Autodesk Fusion 360 part; units mm, degrees
sketch "Skizze1" plane through (0, 0, 0) normal (0, 0, 1) x (1, 0, 0)
  line L0 (-50, 50) -> (0, 50)
  line L1 (0, 50) -> (0, 0)
  line L2 (0, 0) -> (-50, 0)
  line L3 (-50, 0) -> (-50, 50)
  line L4 (-50, 25) -> (0, 25) construction
  line L5 (-25, 50) -> (-25, 0) construction
  circle A0 centre (-25, 25) radius 16.5
  circle A1 centre (-8.0294, 8.0294) radius 3.55
  line L6 (-50, 50) -> (0, 0) construction
  line L7 (0, 50) -> (-50, 0) construction
  circle A2 centre (-43.3848, 43.3848) radius 1.9
  circle A3 centre (-6.6152, 43.3848) radius 1.9
  circle A4 centre (-43.3848, 6.6152) radius 1.9
  line L8 (-6.8665, 50) -> (0, 43.1335)
  line L9 (-50, 6.8665) -> (-43.1335, 0)
  line L10 (-43.1335, 50) -> (-50, 43.1335)
  line L11 (0, 6.8665) -> (-6.8665, 0)
  line L12 (-8.0294, 16.5147) -> (-16.5147, 8.0294) construction
  line L13 (-16.5147, 8.0294) -> (-8.0294, -0.4558) construction
  line L14 (-8.0294, -0.4558) -> (0.4558, 8.0294) construction
  line L15 (0.4558, 8.0294) -> (-8.0294, 16.5147) construction
  line L16 (-8.0294, 16.5147) -> (-8.0294, -0.4558) construction
  point P0 (-8.0294, 8.0294)
  point P1 (-8.0294, 8.0294)
  dimension "d3" = 33
  dimension "d4" = 7.1
  dimension "d6" = 3.8
  dimension "d7" = 26
  dimension "d8" = 26
  dimension "d9" = 26
  dimension "d42" = 50
  dimension "d43" = 50
  dimension "d44" = 61
  dimension "d45" = 61
  dimension "d46" = 12
  dimension "d47" = 12
  dimension "d54" = 6.5
extrude "Extrusion1" add sketch "Skizze1" along normal blind 3 contours L0 L1 L2 L3 L8 L9 L10 L11
chamfer "Fase1" distance 0.8 angle 45 8 edges at (-25, 0, 3) (-46.5668, 3.4332, 3) (-50, 25, 3) (-46.5668, 46.5668, 3) (-25, 50, 3) (-3.4332, 46.5668, 3) (0, 25, 3) (-3.4332, 3.4332, 3)
chamfer "Fase3" distance 2 distance2 1 1 edges at (-40.3834, 30.9667, 3) measured on face at (-24.589, 46.618, 3)
sketch "Skizze2" plane through (0, 0, 0) normal (0, 0, -1) x (1, 0, 0)
  circle A0 centre (-25, -25) radius 16.5
  circle A1 centre (-43.3848, -43.3848) radius 1.9
  circle A2 centre (-43.3848, -6.6152) radius 1.9
  circle A3 centre (-8.0294, -8.0294) radius 3.55
  circle A4 centre (-6.6152, -43.3848) radius 1.9
  line L0 (-50, -43.1335) -> (-43.1335, -50)
  line L1 (-43.1335, -50) -> (-6.8665, -50)
  line L2 (-6.8665, -50) -> (0, -43.1335)
  line L3 (0, -43.1335) -> (0, -6.8665)
  line L4 (0, -6.8665) -> (-6.8665, 0)
  line L5 (-6.8665, 0) -> (-43.1335, 0)
  line L6 (-43.1335, 0) -> (-50, -6.8665)
  line L7 (-50, -6.8665) -> (-50, -43.1335)
  circle A5 centre (-25, -25) radius 18.35
  line L8 (-14.75, -9.7796) -> (-17.9, -3.55)
  line L9 (-17.9, -3.55) -> (-32.1, -3.55)
  line L10 (-32.1, -3.55) -> (-35.25, -9.7796)
  line L11 (-25, -25) -> (-25, 4.0219) construction
  dimension "d18" = 36.7
  dimension "d19" = 21.45
  dimension "d20" = 20.5
  dimension "d21" = 14.2
extrude "Extrusion2" cut sketch "Skizze2" against normal blind 1.5 contours A5 | A5 L8 L9 L10
sketch "Skizze3" plane through (0, 0, 0) normal (0, -1, 0) x (1, 0, 0)
  line L0 (-6.8665, 2.2) -> (-43.1335, 2.2)
  line L1 (-43.1335, 2.2) -> (-43.1335, 0)
  line L2 (-43.1335, 0) -> (-6.8665, 0)
  line L3 (-6.8665, 0) -> (-6.8665, 2.2)
  line L4 (-41.5, 1.5) -> (-8.5, 1.5)
  line L5 (-41.5, 2) -> (-8.5, 2)
  line L6 (-25, 1.5) -> (-25, -10) construction
  line L7 (-22.9, -6.8) -> (-27.1, -6.8)
  line L8 (-22.9, -0.8) -> (-27.1, -0.8)
  arc A0 (-27.1, -0.8) -> (-27.1, -6.8) centre (-27.1, -3.8) ccw
  arc A1 (-22.9, -6.8) -> (-22.9, -0.8) centre (-22.9, -3.8) ccw
  line L9 (-19.9, -3.8) -> (-30.1, -3.8) construction
  line L10 (-25, -5.5) -> (-25, -2.1) construction
  line L11 (-22.9, -6.8) -> (-19.9, -6.8)
  line L12 (-19.9, -6.8) -> (-19.9, -3.8)
  line L13 (-27.1, -6.8) -> (-30.1, -6.8)
  line L14 (-30.1, -6.8) -> (-30.1, -3.8)
  line L15 (-30.1, -6.8) -> (-19.9, -6.8)
  line L16 (-19.9, -6.8) -> (-19.9, -8.8)
  line L17 (-19.9, -8.8) -> (-30.1, -8.8)
  line L18 (-30.1, -8.8) -> (-30.1, -6.8)
  point P0 (-25, -2.1)
  point P1 (-25, -5.5)
  point P2 (-25, -3.8)
  point P3 (-25, -3.8)
  dimension "d24" = 3.6
  dimension "d25" = 7
  dimension "d27" = 6
  dimension "d31" = 10.2
  dimension "d53" = 2
extrude "Extrusion3" add 1 faces at (-47.7677, 25.4366, 0) along direction (0, 0, -1) blind 7
extrude "Extrusion4" cut sketch "Skizze3" against normal up to surface (3.55 mm away) contours L7 L11 L13 L15 L16 L17 L18 | L7 L8 A0 A1 L15 | A1 L11 L12 L15 | A0 L13 L14 L15
sketch "Skizze4" plane through (0, 0, -7) normal (0, 0, -1) x (1, 0, 0)
  circle A0 centre (-43.3848, -43.3848) radius 1.9
  circle A1 centre (-6.6152, -43.3848) radius 1.9
  arc A2 (-35.25, -9.7796) -> (-14.75, -9.7796) centre (-25, -25) ccw
  arc A3 (-35.25, -9.7796) -> (-14.75, -9.7796) centre (-25, -25) ccw
  circle A4 centre (-8.0294, -8.0294) radius 3.55
  circle A5 centre (-8.0294, -8.0294) radius 3.55
  circle A6 centre (-43.3848, -6.6152) radius 1.9
  circle A7 centre (-8.0294, -8.0294) radius 3.5
  circle A8 centre (-8.0294, -8.0294) radius 5
  circle A9 centre (-6.6152, -43.3848) radius 1.1
  circle A10 centre (-6.6152, -43.3848) radius 3
  circle A11 centre (-43.3848, -43.3848) radius 1.1
  circle A12 centre (-43.3848, -43.3848) radius 3
  circle A13 centre (-43.3848, -6.6152) radius 1.1
  circle A14 centre (-43.3848, -6.6152) radius 3
  circle A15 centre (-43.3848, -43.3848) radius 1.9
  circle A16 centre (-6.6152, -43.3848) radius 1.9
  circle A17 centre (-43.3848, -6.6152) radius 1.9
  dimension "d49" = 6
  dimension "d50" = 10
extrude "Extrusion5" cut sketch "Skizze4" against normal blind 4 contours A10 | A12 | A14
extrude "Extrusion6" cut sketch "Skizze4" against normal blind 3 contours A8
sketch "Skizze5" plane through (0, 0, 3) normal (0, 0, 1) x (-1, 0, 0)
  line L0 (7.1979, -49.2) -> (42.8021, -49.2)
  line L1 (42.8021, -49.2) -> (49.2, -42.8021)
  line L2 (49.2, -42.8021) -> (49.2, -7.1979)
  line L3 (49.2, -7.1979) -> (42.8021, -0.8)
  line L4 (42.8021, -0.8) -> (7.1979, -0.8)
  line L5 (7.1979, -0.8) -> (0.8, -7.1979)
  line L6 (0.8, -7.1979) -> (0.8, -42.8021)
  line L7 (0.8, -42.8021) -> (7.1979, -49.2)
  circle A0 centre (43.3848, -43.3848) radius 1.9
  circle A1 centre (43.3848, -6.6152) radius 1.9
  circle A2 centre (6.6152, -43.3848) radius 1.9
  circle A3 centre (8.0294, -8.0294) radius 3.55
  circle A4 centre (25, -25) radius 18.5
  circle A5 centre (6.6152, -43.3848) radius 1.9
  circle A6 centre (6.6152, -43.3848) radius 1.9
  circle A7 centre (43.3848, -43.3848) radius 1.9
  circle A8 centre (43.3848, -43.3848) radius 1.9
  circle A9 centre (43.3848, -6.6152) radius 1.9
  circle A10 centre (43.3848, -6.6152) radius 1.9
  circle A11 centre (43.3848, -43.3848) radius 3.5
  circle A12 centre (43.3848, -6.6152) radius 3.5
  circle A13 centre (6.6152, -43.3848) radius 3.5
  dimension "d55" = 7
extrude "Extrusion7" cut sketch "Skizze5" against normal blind 2.4 contours A11 | A12 | A13
sketch "Skizze6" plane through (0, 0, -7) normal (0, 0, -1) x (1, 0, 0)
  circle A0 centre (-8.0294, -8.0294) radius 5
  line L0 (-30.1, -3.55) -> (-30.1, 0)
  line L1 (-30.1, 0) -> (-43.1335, 0)
  line L2 (-43.1335, 0) -> (-50, -6.8665)
  line L3 (-50, -6.8665) -> (-50, -43.1335)
  line L4 (-50, -43.1335) -> (-43.1335, -50)
  line L5 (-43.1335, -50) -> (-6.8665, -50)
  line L6 (-6.8665, -50) -> (0, -43.1335)
  line L7 (0, -43.1335) -> (0, -6.8665)
  line L8 (0, -6.8665) -> (-6.8665, 0)
  line L9 (-6.8665, 0) -> (-19.9, 0)
  line L10 (-19.9, 0) -> (-19.9, -3.55)
  line L11 (-19.9, -3.55) -> (-17.9, -3.55)
  line L12 (-17.9, -3.55) -> (-14.75, -9.7796)
  arc A1 (-35.25, -9.7796) -> (-14.75, -9.7796) centre (-25, -25) ccw
  line L13 (-35.25, -9.7796) -> (-32.1, -3.55)
  line L14 (-32.1, -3.55) -> (-30.1, -3.55)
  circle A2 centre (-6.6152, -43.3848) radius 3
  circle A3 centre (-43.3848, -43.3848) radius 3
  circle A4 centre (-43.3848, -6.6152) radius 3
  circle A5 centre (-6.6152, -43.3848) radius 3
  circle A6 centre (-43.3848, -43.3848) radius 3
  circle A7 centre (-43.3848, -6.6152) radius 3
  circle A8 centre (-8.0294, -8.0294) radius 5
  circle A9 centre (-25, -25) radius 19.5
  dimension "d58" = 39
equation "d8 = d7"
equation "d9 = d7"
equation "d54 = 6.85 mm - 0.35 mm"
CAD build for the part. Positions are in the model's coordinates, mm. A direction names the side the tool comes from. Round coordinates to 2 decimals unless told otherwise and drop trailing zeros. Order: outer loops, then holes, each group sorted by start corner. A loop starts at its lowest first (then second) coordinate and runs counter-clockwise, first axis right, second up. Notation, with made-up numbers: (-6.75, 54) -> (49.25, 54) arc R24 ccw to (49.25, 73) -> close; hole circle Ø10 at (32, -29). An arc over 180 degrees is marked (long way). Write item = value, one per line. Start each with the question number.
(1) Cut at C-C, the plane z = -5.5. List the corners of the cut face in (x, y), then the cut area to 3 significant figures.
(2) Cut at B-B, the plane y = 25. List the corners of the cut face in (x, z), then the cut area to 3 significant figures.
(3) Pull direction X, two halves, no side cores. Call faces 4 (the flat face through (-36, 42, -7)), 5 (the flat face through (-46.232, 3.672, 2.606)), 6 (the cylindrical face through (-20.76, 1.75, -1.7)): released by +X, released by -X, zero draft, split by the parting line, or undercut.
(4) Cut at D-D, the plane y = 44.5. State how many separate pieces and enclosed holes the cut face has, then the cut area to 3 significant figures.
(5) Pin check, flat tips, straight feed: P1, Ø2.5, axis at y = 2, z = -5, coming from the -X side; P2, Ø3, axis at x = -43, y = 8, coming from the -Z side; P3, Ø5.5, axis at x = -43.38, y = 43.38, coming from the +Z side. Stop position of each tip, or through.
(6) Which spindle directions (+Z, -Z, +X, -X, +Y, -Y) get a long thin tool onto all of the face, cutting with end or side? Do faces 1 (the cylindrical face through (-42.363, 41.783, -1.225)), 2 (the flat face through (-19.9, 2, -5)), 3 (the flat face through (-4.66, 44.01, -3)). Say none if no direction does.
(7) Probe line 1 (Y direction, x = -5, z = 2); line 2 (Y direction, x = -46, z = -4); line 3 (Y direction, x = -8, z = -4.25). List the from-to ranges inside material, lowest first. Write a range as [from, to].
(8) Cut at A-A, the plane x = -25. List the corners of the cut face in (y, z), then the cut area to 4 significant figures.
Model answer:
q1.outline = (-50, 6.87) -> (-43.13, 0) -> (-30.1, 0) -> (-30.1, 3.55) -> (-32.1, 3.55) -> (-35.25, 9.78) arc R18.35 cw (long way) to (-14.75, 9.78) -> (-17.9, 3.55) -> (-19.9, 3.55) -> (-19.9, 0) -> (-6.87, 0) -> (0, 6.87) -> (0, 43.13) -> (-6.87, 50) -> (-43.13, 50) -> (-50, 43.13) -> close; hole circle Ø6 at (-43.38, 6.62); hole circle Ø6 at (-43.38, 43.38); hole circle Ø10 at (-8.03, 8.03); hole circle Ø6 at (-6.62, 43.38)
q1.area = 1,080 mm2
q2.outline = (-50, -7) -> (-43.35, -7) -> (-43.35, 1.5) -> (-41.5, 1.5) -> (-41.5, 2) -> (-43.5, 3) -> (-49.2, 3) -> (-50, 2.2) -> close; (-8.5, 1.5) -> (-6.65, 1.5) -> (-6.65, -7) -> (0, -7) -> (0, 2.2) -> (-0.8, 3) -> (-6.5, 3) -> (-8.5, 2) -> close
q2.area = 136 mm2
q3.face_4 = zero draft
q3.face_5 = released by -X
q3.face_6 = undercut
q4.separate_pieces = 3
q4.enclosed_holes = 0
q4.area = 373 mm2
q5.P1 = -46.38
q5.P2 = -3
q5.P3 = 0.6
q6.face_1 = +Z, -Z
q6.face_2 = -Z, -Y
q6.face_3 = -Z
q7.line_1 = [1.87, 6.18], [9.88, 40.28], [46.49, 48.13]
q7.line_2 = [2.87, 5.15], [8.09, 41.91], [44.85, 47.13]
q7.line_3 = [0, 3.03], [13.03, 18.09], [31.91, 40.72], [46.05, 50]
q8.outline = (0, -0.8) -> (3.55, -0.8) -> (3.55, 1.5) -> (8.5, 1.5) -> (8.5, 2) -> (6.5, 3) -> (0.8, 3) -> (0, 2.2) -> close; (41.5, 1.5) -> (43.35, 1.5) -> (43.35, -7) -> (50, -7) -> (50, 2.2) -> (49.2, 3) -> (43.5, 3) -> (41.5, 2) -> close
q8.area = 87.55 mm2
